```python
from build123d import *

# Parameters (mm, degrees)
F0_R     = 4.000037
F0_R_2   = 4
F1_DEPTH = 10


with BuildPart() as f1:
    # F0 (on Front) → F1 (new body)
    with BuildSketch(Plane.XZ):
        with BuildLine():
            Line((-53.562295, 17.812143), (-39.631873, 17.812143))
            Line((-39.631873, 17.812143), (-39.631873, 22.812143))
            Line((-39.631873, 22.812143), (-59.631873, 22.812143))
            Line((-59.631873, 22.812143), (-59.631873, 12.812143))
            Line((-59.631873, 12.812143), (-66.560792, 12.812143))
            ThreePointArc((-66.560792, 12.812143), (-94.406932, 11.300926), (-66.738905, 7.812143))
            Line((-66.738905, 7.812143), (-59.631873, 7.812143))
            Line((-59.631873, 7.812143), (-59.631873, -2.187857))
            Line((-59.631873, -2.187857), (-39.631873, -2.187857))
            Line((-39.631873, -2.187857), (-39.631873, 2.812143))
            Line((-39.631873, 2.812143), (-53.562295, 2.812143))
            Line((-53.562295, 2.812143), (-53.562295, 7.812143))
            Line((-53.562295, 7.812143), (-39.631873, 7.812143))
            Line((-39.631873, 7.812143), (-34.631873, 7.812143))
            Line((-34.631873, 7.812143), (-34.631873, -2.187857))
            Line((-34.631873, -2.187857), (-29.631873, -2.187857))
            Line((-29.631873, -2.187857), (-29.631873, 7.812143))
            Line((-29.631873, 7.812143), (-24.631873, 7.812143))
            Line((-24.631873, 7.812143), (-24.631873, -2.187857))
            Line((-24.631873, -2.187857), (-19.631873, -2.187857))
            Line((-19.631873, -2.187857), (-12.131873, 10.802524))
            Line((-12.131873, 10.802524), (-2.131873, 10.802524))
            Line((-2.131873, 10.802524), (5.368127, -2.187857))
            Line((5.368127, -2.187857), (10.368127, -2.187857))
            Line((10.368127, -2.187857), (10.368127, 13.015858))
            Line((10.368127, 13.015858), (19.145996, -2.187857))
            Line((19.145996, -2.187857), (24.145996, -2.187857))
            Line((24.145996, -2.187857), (24.145996, 7.406078))
            Line((24.145996, 7.406078), (27.516475, 7.406078))
            ThreePointArc((27.516475, 7.406078), (55.093287, 11.174656), (27.35517, 13.472397))
            Line((27.35517, 13.472397), (24.145996, 13.472397))
            Line((24.145996, 13.472397), (24.145996, 22.132651))
            Line((24.145996, 22.132651), (20.368127, 22.132651))
            Line((20.368127, 22.132651), (20.368127, 4.812143))
            Line((20.368127, 4.812143), (10.368127, 22.132651))
            Line((10.368127, 22.132651), (5.368127, 22.132651))
            Line((5.368127, 22.132651), (5.368127, 6.907172))
            Line((5.368127, 6.907172), (5.368127, 4.812143))
            Line((5.368127, 4.812143), (-4.631873, 22.132651))
            Line((-4.631873, 22.132651), (-9.631873, 22.132651))
            Line((-9.631873, 22.132651), (-19.631873, 4.812143))
            Line((-19.631873, 4.812143), (-19.631873, 6.907172))
            Line((-19.631873, 6.907172), (-19.631873, 24.812143))
            Line((-19.631873, 24.812143), (-9.631873, 24.812143))
            Line((-9.631873, 24.812143), (-9.631873, 29.812143))
            Line((-9.631873, 29.812143), (-34.631873, 29.812143))
            Line((-34.631873, 29.812143), (-34.631873, 24.812143))
            Line((-34.631873, 24.812143), (-24.631873, 24.812143))
            Line((-24.631873, 24.812143), (-24.631873, 12.812143))
            Line((-24.631873, 12.812143), (-29.631873, 12.812143))
            Line((-29.631873, 12.812143), (-29.631873, 22.812143))
            Line((-29.631873, 22.812143), (-34.631873, 22.812143))
            Line((-34.631873, 22.812143), (-34.631873, 12.812143))
            Line((-34.631873, 12.812143), (-39.631873, 12.812143))
            Line((-39.631873, 12.812143), (-53.562295, 12.812143))
            Line((-53.562295, 12.812143), (-53.562295, 17.812143))
        make_face()
        with BuildLine():
            ThreePointArc((-73.200306, 6.85316), (-80.415806, -0.36234), (-87.631306, 6.85316))
            Line((-87.631306, 6.85316), (-73.200306, 6.85316))
        make_face(mode=Mode.SUBTRACT)
        with BuildLine():
            ThreePointArc((48.313583, 6.85316), (41.098233, -0.36219), (33.882884, 6.85316))
            Line((33.882884, 6.85316), (48.313583, 6.85316))
        make_face(mode=Mode.SUBTRACT)
        with Locations((-85.42119, 15.723815)):
            Circle(F0_R, mode=Mode.SUBTRACT)
        with Locations((-74.859366, 15.723815)):
            Circle(F0_R_2, mode=Mode.SUBTRACT)
        Polygon((-9.631873, 17.345985), (-4.631873, 17.345985), (-2.131873, 13.015858), (-12.131873, 13.015858), align=None, mode=Mode.SUBTRACT)
        with Locations((35.980549, 15.723815)):
            Circle(F0_R_2, mode=Mode.SUBTRACT)
        with Locations((46.898279, 15.723815)):
            Circle(F0_R_2, mode=Mode.SUBTRACT)
    extrude(amount=F1_DEPTH)


solid = f1.part
```
Can you work these out from the model? Positions are in its coordinate system, mm. A direction names the side the tool comes from. Coordinates: 2 decimals unless noted, no trailing zeros. Order: outer loops, then holes, each group sorted by start corner. A loop starts at its lowest first (then second) coordinate and runs counter-clockwise, first axis right, second up. Notation, with made-up numbers: (-3, 83) - (2, 83) arc R4 ccw to (2, 90) - close; hole circle Ø4 at (31, 29.25). An arc over 180 degrees is marked (long way). Answer in a Markdown table with one row per item.
1. Suppose I cut it at D-D (x = 17). Please give me the cut outline in (y, z), and give its area (3 significant figures).
Reply:
| item | result |
|---|---|
| outline | (-10, 1.53) - (0, 1.53) - (0, 10.65) - (-10, 10.65) - close |
| area | 91.2 mm^2 |
2. For pin 1 (1.5 mm diameter, centred on y = -2.5, z = 16, fed in from +X); pin 2 (3 mm diameter, centred on x = -43.5, y = -3, fed in from +Z); pin 3 (2 mm diameter, centred on x = -63, y = -4, fed in from -Z), each with a flat end and sliding along its axis, tell me the tip position at first contact or that it passes through.
Reply:
| item | result |
|---|---|
| pin 1 | stops at x = 54.37 |
| pin 2 | stops at z = 22.81 |
| pin 3 | stops at z = 7.81 |
3. Suppose I cut it at C-C (y = -6.25). Give the number of separate pieces and of enclosed holes in the cut face, and give its area (3 significant figures).
Reply:
| item | result |
|---|---|
| separate pieces | 1 |
| enclosed holes | 7 |
| area | 2,190 mm^2 |
4. Suppose I cut it at B-B (x = -84). Please give me the cut outline in (y, z).
Reply:
| item | result |
|---|---|
| outline | (-10, -2.73) - (0, -2.73) - (0, 0.59) - (-10, 0.59) - close; (-10, 6.85) - (0, 6.85) - (0, 11.98) - (-10, 11.98) - close; (-10, 19.46) - (0, 19.46) - (0, 24.34) - (-10, 24.34) - close |
5. For faces 1 (the flat face through (-81, -5, 6.853)), 2 (the flat face through (-7, -5, 22.133)), 3 (the flat face through (-27, -5, 7.812)), which set-ups out of +Z, -Z, +X, -X, +Y, -Y let a thin tool reach every point of the face, with its end or its side?
Reply:
| item | result |
|---|---|
| face 1 | +Y, -Y |
| face 2 | +Z, +Y, -Y |
| face 3 | -Z, +Y, -Y |
6. If I drill on line 1 along Z through (x, y) = (-50, -6.75); line 2 along Z through (x, y) = (47.5, -0.75); line 3 along Z through (x, y) = (-26.5, -7.5), over which ranges is the centre line in solid material (lowest first)?
Reply:
| item | result |
|---|---|
| line 1 | z = -2.19 to 2.81, 7.81 to 12.81, 17.81 to 22.81 |
| line 2 | z = -1.65 to 3.52, 6.85 to 11.77, 19.68 to 23.25 |
| line 3 | z = 7.81 to 12.81, 24.81 to 29.81 |
7. Suppose I cut it at A-A (x = -46). Please give me the cut outline in (y, z), and give its area (3 significant figures).
Reply:
| item | result |
|---|---|
| outline | (-10, -2.19) - (0, -2.19) - (0, 2.81) - (-10, 2.81) - close; (-10, 7.81) - (0, 7.81) - (0, 12.81) - (-10, 12.81) - close; (-10, 17.81) - (0, 17.81) - (0, 22.81) - (-10, 22.81) - close |
| area | 150 mm^2 |
